Autodesk Inventor part; units mm, degrees
ref_plane "YZ Plane" through (0, 0, 0) normal (1, 0, 0) x (0, 1, 0)
ref_plane "XZ Plane" through (0, 0, 0) normal (0, 1, 0) x (-1, 0, 0)
ref_plane "XY Plane" through (0, 0, 0) normal (0, 0, 1) x (1, 0, 0)
sketch "Sketch1" plane through (0, 0, 0) normal (0, 1, 0) x (-1, 0, 0)
  line L0 (0, -37.4904) -> (0, 6.2484)
  line L1 (-44.958, 0) -> (7.493, 0)
  line L2 (0, 0) -> (-37.465, 0)
  line L3 (-37.465, 0) -> (-37.465, -9.525)
  line L4 (-37.465, -9.525) -> (0, -9.525)
  line L5 (0, -9.525) -> (0, 0)
  line L6 (0, -9.525) -> (-12.7, -9.525)
  line L7 (-12.7, -9.525) -> (-12.7, -31.242)
  line L8 (0, -31.242) -> (0, -9.525)
  line L9 (0, -31.242) -> (-12.7, -31.242)
  dimension "d10" = 9.525
  dimension "d36" = 31.242
  dimension "d37" = 12.7
  dimension "d38" = 37.465
extrude "Extrusion3" add sketch "Sketch1" along normal mid plane 41.91
sketch "Sketch2" plane through (37.465, 20.955, -9.525) normal (0, 0, -1) x (-1, 0, 0)
  line L0 (24.765, -41.91) -> (24.765, 0)
  line L1 (0, 0) -> (24.765, 0)
  line L2 (0, -41.91) -> (0, 0)
  line L3 (24.765, -41.91) -> (0, -41.91)
  line L4 (-7.493, -20.955) -> (44.958, -20.955)
  line L5 (37.465, -41.91) -> (37.465, 0)
  point P0 (37.465, -20.955)
  point P1 (15.875, -20.955)
  dimension "d56" = 0
  dimension "d57" = 21.59
hole "Hole1" at (21.59, 0, -9.525) direction (0, 0, 1) diameter 5.5118 end through all
sketch "Sketch3" plane through (0, -20.955, 0) normal (0, 1, 0) x (-1, 0, 0)
  line L0 (-12.7, -31.242) -> (-12.7, -9.525)
  line L1 (-12.7, -9.525) -> (-37.465, -9.525)
  line L2 (-37.465, -9.525) -> (-12.7, -31.242)
  line L3 (-12.7, -31.242) -> (-12.7, -9.525)
  line L4 (-37.465, -9.525) -> (-12.7, -9.525)
  point P0 (0, 0)
extrude "Extrusion4" add sketch "Sketch3" along normal blind 6.35
sketch "Sketch4" plane through (12.7, 20.955, -31.242) normal (0, 0, -1) x (-1, 0, 0)
  line L0 (12.7, -50.292) -> (12.7, 8.382)
  line L1 (-32.258, -20.955) -> (20.193, -20.955)
  line L2 (0, -35.56) -> (0, 0)
  point P0 (12.7, -20.955)
  point P1 (6.35, -9.525)
  point P2 (6.35, -32.385)
  point P3 (6.35, -20.955)
  dimension "d39" = 11.43
  dimension "d40" = 11.43
  dimension "d41" = 6.35
  dimension "d63" = 12.7
hole "Hole2" at (6.35, 11.43, -31.242) at (6.35, -11.43, -31.242) at (6.35, 0, -31.242) direction (0, 0, 1) diameter 2.4384 depth 10.16 tip angle 118
sketch "Sketch5" plane through (12.7, 20.955, -9.525) normal (1, 0, 0) x (0, 0, -1)
  line L0 (-15.7734, -20.955) -> (27.9654, -20.955)
  line L1 (-9.525, -50.292) -> (-9.525, 8.382)
  line L2 (14.097, -12.0015) -> (15.875, -12.0015)
  line L3 (15.875, -12.0015) -> (15.875, -7.0485)
  line L4 (15.875, -7.0485) -> (14.097, -7.0485)
  line L5 (14.097, -7.0485) -> (14.097, -12.0015)
  line L6 (14.097, -12.0015) -> (15.875, -7.0485) construction
  line L7 (15.875, -12.0015) -> (14.097, -7.0485) construction
  line L8 (14.097, -23.4315) -> (15.875, -23.4315)
  line L9 (15.875, -23.4315) -> (15.875, -18.4785)
  line L10 (15.875, -18.4785) -> (14.097, -18.4785)
  line L11 (14.097, -18.4785) -> (14.097, -23.4315)
  line L12 (14.097, -23.4315) -> (15.875, -18.4785) construction
  line L13 (15.875, -23.4315) -> (14.097, -18.4785) construction
  line L14 (14.097, -34.8615) -> (15.875, -34.8615)
  line L15 (15.875, -34.8615) -> (15.875, -29.9085)
  line L16 (15.875, -29.9085) -> (14.097, -29.9085)
  line L17 (14.097, -29.9085) -> (14.097, -34.8615)
  line L18 (14.097, -34.8615) -> (15.875, -29.9085) construction
  line L19 (15.875, -34.8615) -> (14.097, -29.9085) construction
  line L20 (21.717, -35.56) -> (21.717, 0)
  point P0 (-9.525, -20.955)
  point P1 (14.986, -9.525)
  point P2 (14.986, -20.955)
  point P3 (14.986, -32.385)
  point P4 (14.986, -9.525)
  point P5 (14.986, -32.385)
  dimension "d49" = 4.953
  dimension "d50" = 1.778
  dimension "d51" = 11.43
  dimension "d58" = 7.62
  dimension "d59" = 11.43
extrude "Extrusion5" cut sketch "Sketch5" along normal blind 10.16 and the other way blind 8.89
sketch "Sketch6" plane through (0, 20.955, 0) normal (0, 1, 0) x (1, 0, 0)
  line L0 (12.7, 9.525) -> (12.7, 31.242)
  line L1 (37.465, 9.525) -> (12.7, 9.525)
  line L2 (37.465, 9.525) -> (12.7, 31.242)
  point P0 (0, 0)
extrude "Extrusion6" add sketch "Sketch6" against normal blind 6.35
sketch "Sketch7" plane through (0, 20.955, 0) normal (0, 1, 0) x (1, 0, 0)
  line L0 (0, 0) -> (37.465, 0)
  line L1 (37.465, 0) -> (37.465, 9.525)
  line L2 (25.7746, 0) -> (37.5697, -3.1605)
  line L3 (37.5697, -3.1605) -> (37.465, 0)
  line L4 (25.7746, 0) -> (37.465, 0)
  dimension "d64" = 11.684
  dimension "d65" = 15
extrude "Extrusion7" [suppressed]
sketch "Sketch8" plane through (37.465, -20.955, 0) normal (1, 0, 0) x (0, 0, -1)
  line L0 (9.525, 0) -> (9.525, 6.35)
  line L1 (9.525, 6.35) -> (9.525, 35.56)
  line L2 (9.525, 35.56) -> (9.525, 41.91)
  line L3 (0, 41.91) -> (9.525, 41.91)
  line L4 (0, 0) -> (0, 41.91)
  line L5 (9.525, 0) -> (0, 0)
  line L6 (9.525, 41.91) -> (-3.81, 41.91)
  line L7 (-3.81, 41.91) -> (-3.81, 0)
  line L8 (-3.81, 0) -> (9.525, 0)
  line L9 (9.525, 0) -> (9.525, 41.91)
  point P0 (0, 20.955)
  dimension "d68" = 0
  dimension "d69" = 3.81
extrude "Extrusion8" add sketch "Sketch8" along normal blind 3.81
fillet "Fillet2" radius 3.175 4 edges at (37.465, 17.78, -9.525) (37.465, -17.78, -9.525) (39.37, 20.955, 3.81) (39.37, -20.955, 3.81)
properties material "ABS, BLACK"
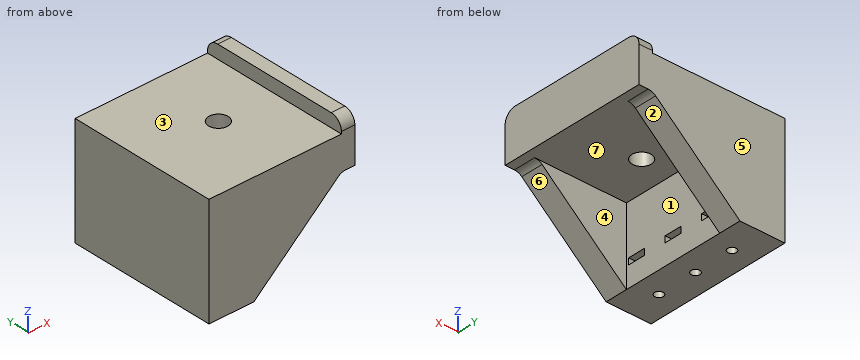
Verification items for the finished model (mm, model axes). Face numbers are marked on the shaded views. A direction names the side the tool comes from. Coordinates: 2 decimals unless noted, no trailing zeros. Write each loop counter-clockwise with the first axis right and the second up, starting at its lowest first coordinate (ties: lowest second). Pieces come first, ordered by that corner, then holes. Notation, with made-up numbers: M 64.25,29.25 L 73.25,29.25 A34 ccw 73.25,60.25 Z; hole C 11,25.25 d1. An arc over 180 degrees is marked long. One line per item, written item: value.
Item 1: Section check A-A, the plane x = 12. Record the boundary of the cut face in (y, z) (1 decimal), plus the area to 3 significant figures.
Check sheet entries:
outline: M -21,-31.2 L 21,-31.2 L 21,0 L -21,0 Z; hole M -13.9,-25.4 L -9,-25.4 L -9,-23.6 L -13.9,-23.6 Z; hole M -2.5,-25.4 L 2.5,-25.4 L 2.5,-23.6 L -2.5,-23.6 Z; hole M 9,-25.4 L 13.9,-25.4 L 13.9,-23.6 L 9,-23.6 Z
area: 1,280 mm^2
Item 2: Scan lines: line 1 along X through (y, z) = (11.43, -21.7); line 2 along Y through (x, z) = (30, -10.5) (3 decimals); line 3 along X through (y, z) = (0, -5) (3 decimals). Record each from-to range of solid material in increasing order.
Check sheet entries:
line 1: x = 0 to 5.13, 7.57 to 12.7
line 2: y = -20.955 to -14.605, 14.605 to 20.955
line 3: x = 0 to 18.834, 24.346 to 41.275
Item 3: Section check C-C, the plane x = 20.5. Record the boundary of the cut face in (y, z) (3 decimals), plus the area to 3 significant figures.
Check sheet entries:
outline: M -20.955,-24.402 L -14.605,-24.402 L -14.605,-9.525 L -2.531,-9.525 L -2.531,0 L -20.955,0 Z; M 2.531,-9.525 L 14.605,-9.525 L 14.605,-24.402 L 20.955,-24.402 L 20.955,0 L 2.531,0 Z
area: 540 mm^2
Item 4: Section check D-D, the plane z = -22.5. Record the boundary of the cut face in (x, y) (3 decimals).
Check sheet entries:
outline: M 0,-20.955 L 22.669,-20.955 L 22.669,-14.605 L 12.7,-14.605 L 12.7,14.605 L 22.669,14.605 L 22.669,20.955 L 0,20.955 Z; hole C 6.35,-11.43 d2.438; hole C 6.35,0 d2.438; hole C 6.35,11.43 d2.438
Item 5: Gauge pin test, flat ends, axial feed: pin 1 Ø8.5 at (x, y) = (29, 9) entering from -Z (3 decimals); pin 2 Ø8 at (x, y) = (14, 6) entering from +Z; pin 3 Ø0.5 at (y, z) = (11, -25) entering from +X. Record the tip position at first contact, or that the pin passes through.
Check sheet entries:
pin 1: stops at z = -9.525
pin 2: stops at z = 0
pin 3: stops at x = 3.81
Item 6: Access from +Z, -Z, +X, -X, +Y, -Y to the whole of each face (thin tool, end or side, straight path). Record for the marked faces 1, 2 and 3.
Check sheet entries:
face 1: -Z, +X
face 2: -Z, +X, +Y, -Y
face 3: +Z, -X, +Y, -Y
Item 7: Section check B-B, the plane y = 8. Record the boundary of the cut face in (x, z) (3 decimals), plus the area to 3 significant figures.
Check sheet entries:
outline: M 0,-31.242 L 12.7,-31.242 L 12.7,-9.525 L 41.275,-9.525 L 41.275,3.81 L 37.465,3.81 L 37.465,0 L 0,0 Z
area: 683 mm^2
Item 8: Mould release check, pull along Y, two halves, no side actions. Record for the marked faces 4, 5, 6 and 7: pulls with the +Y half, pulls with the -Y half, needs draft (parallel to the pull), parting line crosses it, or undercut.
Check sheet entries:
face 4: undercut
face 5: pulls with the +Y half
face 6: needs draft
face 7: undercut
